Read the model definition and answer for the solid it produces. Units are mm, in the model's axes. A direction names the side the tool comes from. Round coordinates to 2 decimals unless told otherwise and drop trailing zeros. Use one line per item in the form item = value. Start each with the question number.
```python
from build123d import *

# Parameters (mm, degrees)
F0_R     = 15
F1_DEPTH = 10
F3_R     = 13.4495
F4_DEPTH = 4
F5_W     = 6
F5_H     = 6
F6_DEPTH = 3
F7_R     = 1.75
F8_DEPTH = 1.5


# Not quite as in the source:
# - a fillet or chamfer that OpenCascade refuses, or shapes differently, is made with other operations: its cross-section is extruded or revolved along the edge and cut away or added


with BuildPart() as f1:
    # F0 (on Top) → F1 (new body)
    with BuildSketch(Plane.XY):
        Circle(F0_R)
    extrude(amount=F1_DEPTH)

    # F2: fillet of radius 15 on 1 edges, made by hand

    # F2_s1 → F2_t2 (revolve, cut)
    with BuildSketch(Plane.XZ):
        with BuildLine():
            ThreePointArc((15, 0), (9.5181184141, 7.2474487139), (0.8578643763, 10))
            Line((0.8578643763, 10), (15, 10))
            Line((15, 10), (15, 0))
        make_face()
    revolve(axis=Axis((0, 0, 10), (0, 0, 1)), mode=Mode.SUBTRACT)

    # F3 (on face) → F4 (join)
    with BuildSketch(Plane(origin=(0, 0, 0), x_dir=(1, 0, 0), z_dir=(0, 0, -1))):
        Circle(F3_R)
    extrude(amount=F4_DEPTH)

    # F5 (on face) → F6 (cut)
    with BuildSketch(Plane(origin=(0, 0, -4), x_dir=(1, 0, 0), z_dir=(0, 0, -1))):
        Rectangle(F5_W, F5_H)
    extrude(amount=-F6_DEPTH, mode=Mode.SUBTRACT)

    # F7 (on face) → F8 (cut)
    with BuildSketch(Plane(origin=(0, 0, -1), x_dir=(1, 0, 0), z_dir=(0, 0, -1))):
        Circle(F7_R)
    extrude(amount=-F8_DEPTH, mode=Mode.SUBTRACT)


solid = f1.part
```
Q1. Straight lines are drawn through the part: line 1 (X direction, y = 0, z = -0.55); line 2 (Y direction, x = -1, z = -2.25). For each, find the intervals that lie inside material, in ascending order. Write a range as [from, to].
Q2. Each of these flat-tipped pins is pushed along its axis until it touches: pin 1 Ø3.5 at (x, z) = (-1.5, -2) entering from +Y; pin 2 Ø2.5 at (x, z) = (0, -3) entering from -Y; pin 3 Ø2 at (y, z) = (-2.5, -0.5) entering from +X. Where does it stop, or does it pass through?
Q3. A tool of negligible diameter and unlimited length cuts with its end or side. For faces 4 (the face through (-0.2, -3.2, -4)), 5 (the face through (0, 3, -3)), from which of +Z, -Z, +X, -X, +Y, -Y can it reach the whole face along a straight path? Write none if from no direction.
Q4. For a pull along X with two mould halves and no side action, classify faces 1 (the face through (-9.91, -9.09, -1.97)), 2 (the face through (-3.4, 13.4, 0)), 3 (the face through (1.3, -1.4, -1)) as +X half, -X half, draft (parallel to the pull), parting line (faces both ways), or undercut.
Response:
q1.line_1 = [-13.45, -1.75], [1.75, 13.45]
q1.line_2 = [-13.41, -3], [3, 13.41]
q2.pin_1 = 13.45
q2.pin_2 = -13.45
q2.pin_3 = 14.91
q3.face_4 = -Z, +X, -X, +Y, -Y
q3.face_5 = -Z
q4.face_1 = parting line
q4.face_2 = draft
q4.face_3 = undercut
